from build123d import *

# Parameters (mm, degrees)
F1_DEPTH = 2.54
F3_D     = 6.7564
F4_R     = 5.08
F5_R     = 5.08
F7_D     = 3
F9_D     = 3


with BuildPart() as f1:
    # F0 (on Top) → F1 (new body)
    with BuildSketch(Plane.XY):
        Polygon((-46.2908484042, 37.6848205924), (-45.9911487997, 24.9666236341), (-29.9353669436, 24.9666236341), (-29.9353669436, 16.4984129369), (-45.6991419196, 16.4984129369), (-45.9911487997, 4.7181551345), (-29.9353669436, 4.3201673446), (-10.0788730235, 4.3201673446), (-10.0788730235, 24.9666236341), (46.2785349189, 25.2586323768), (46.2785349189, 37.8149449825), (-30.5147636682, 37.8149449825), align=None)
    extrude(amount=F1_DEPTH)

    # F3 (through all)
    with Locations(Plane.XY.offset(2.54)):
        with Locations((-20.0071199835, 21.1749691516)):
            Hole(F3_D / 2)

    # F4
    f4_edges = [f1.edges().sort_by_distance(p)[0] for p in [
        (-45.991149, 4.718155, 1.27),
    ]]
    fillet(f4_edges, radius=F4_R)

    # F5
    f5_edges = [f1.edges().sort_by_distance(p)[0] for p in [
        (-46.290848, 37.684821, 1.27),
    ]]
    fillet(f5_edges, radius=F5_R)

    # F7 (through all)
    with Locations(Plane.XY.offset(2.54)):
        with Locations((-38.8525593063, 37.7273665891)):
            Hole(F7_D / 2)

    # F9 (through all)
    with Locations(Plane.XY.offset(2.54)):
        with Locations((-38.8401874188, 4.5922716895)):
            Hole(F9_D / 2)


solid = f1.part
Input: part model. Units: mm. Frame: model coordinates. A direction names the side the tool comes from. Give positions to 0.01 mm unless a question says otherwise; leave off trailing zeros. Loops run counter-clockwise (first coordinate to the right, second up) from the corner with the lowest first, then second, coordinate; pieces in that order, holes last. Notation, with made-up numbers: (13, 59.25) - (47, 59.25) arc R24 cw to (47, 90.25) - close; hole circle Ø4 at (-23.75, -9.5). An arc over 180 degrees is marked (long way). Use CSV: the item, a comma, the result in double quotes. Start each with the question number.
Item 1: Section C-C on x = 17.5. Return loops of the section in (y, z), then the cut area to 3 significant figures.
Item 2: Contact query for flat-ended pins moving along their axis: P1, Ø8, axis at x = -4, y = 10, coming from the +Z side; P2, Ø0.8, axis at x = -38.5, z = 1.5, coming from the +Y side; P3, Ø0.8, axis at y = 18.5, z = 1.5, coming from the -X side; P4, Ø8, axis at x = -20.01, y = 21.17, coming from the +Z side. Output: stop coordinate, or through.
Item 3: Mould query, pull axis X, two halves, no side actions, for faces 3 (the cylindrical face through (-38.837, 6.092, 1.252)), 4 (the flat face through (-10.079, 14, 1)), 5 (the flat face through (8, 37.815, 1)). Classes: pulls with the +X half, pulls with the -X half, needs draft (parallel to the pull), parting line crosses it, or undercut.
Item 4: Section A-A on z = 0.9. Return loops of the section in (x, y).
Item 5: Line query: line 1 (Y direction, x = -30, z = 0.95); line 2 (Y direction, x = 42.5, z = 0.2); line 3 (X direction, y = 23, z = 0.55). Output: solid intervals per line, ascending.
Item 6: Section B-B on y = 14.5. Return loops of the section in (x, z).
Item 7: Reachability of faces 1 (the flat face through (-38, 16.498, 1)), 2 (the flat face through (-20, 4.32, 1)) from +Z, -Z, +X, -X, +Y, -Y: full face, straight path, thin tool, end or side. Return the list, or none.
Ans:
1,outline,"(25.11, 0) - (37.81, 0) - (37.81, 2.54) - (25.11, 2.54) - close"
1,area,"32.3 mm2"
2,P1,"passes through"
2,P2,"stops at y = 36.43"
2,P3,"stops at x = -29.94"
2,P4,"stops at z = 2.54"
3,face 3,"undercut"
3,face 4,"pulls with the +X half"
3,face 5,"needs draft"
4,outline,"(-46.17, 32.53) - (-45.99, 24.97) - (-29.94, 24.97) - (-29.94, 16.5) - (-45.7, 16.5) - (-45.87, 9.8) arc R5.08 ccw to (-40.91, 4.59) - (-40.34, 4.58) arc R1.5 cw (long way) to (-37.34, 4.5) - (-29.94, 4.32) - (-10.08, 4.32) - (-10.08, 24.97) - (46.28, 25.26) - (46.28, 37.81) - (-30.51, 37.81) - (-37.35, 37.76) arc R1.5 cw (long way) to (-40.35, 37.73) - (-41.13, 37.73) arc R5.08 ccw to start; hole circle Ø6.76 at (-20.01, 21.17)"
5,line 1,"y = 4.32 to 16.5, 24.97 to 37.81"
5,line 2,"y = 25.24 to 37.81"
5,line 3,"x = -29.94 to -22.85, -17.16 to -10.08"
6,outline,"(-45.75, 0) - (-10.08, 0) - (-10.08, 2.54) - (-45.75, 2.54) - close"
7,face 1,"+Z, -Z, -X"
7,face 2,"+Z, -Z, +X, -X, -Y"
